Autodesk Fusion 360 part; units mm, degrees
sketch "Sketch1" plane through (0, 0, 0) normal (0, 1, 0) x (1, 0, 0)
  line L0 (0, 0) -> (50, 0)
  line L1 (50, 0) -> (50, -30)
  line L2 (50, -30) -> (0, -30)
  line L3 (0, -30) -> (0, 0)
  circle A0 centre (5.5, -15) radius 1.6
  circle A1 centre (44.5, -15) radius 1.6
  circle A2 centre (25, -21.15) radius 2.1
  point P0 (25, -21.15)
  dimension "d1" = 30
  dimension "d2" = 50
  dimension "d3" = 15
  dimension "d4" = 5.5
  dimension "d5" = 5.5
  dimension "d6" = 3.2
  dimension "d9" = 25
  dimension "d10" = 21.15
  dimension "d19" = 4.2
extrude "Extrude1" add sketch "Sketch1" against normal blind 5
sketch "Sketch2" plane through (0, -5, 0) normal (0, -1, 0) x (1, 0, 0)
  circle A0 centre (44.5, 15) radius 1.6
  circle A1 centre (5.5, 15) radius 1.6
  line L0 (50, 30) -> (0, 30)
  line L1 (0, 30) -> (0, 0)
  line L2 (0, 0) -> (50, 0)
  line L3 (50, 0) -> (50, 30)
  line L4 (33.75, 33.4) -> (16.25, 33.4)
  line L5 (16.25, 33.4) -> (16.25, 8.9)
  line L6 (16.25, 8.9) -> (33.75, 8.9)
  line L7 (33.75, 8.9) -> (33.75, 33.4)
  line L8 (33.75, 33.4) -> (16.25, 8.9) construction
  line L9 (16.25, 33.4) -> (33.75, 8.9) construction
  circle A2 centre (25, 21.15) radius 2.1
  line L10 (29.75, 12.9) -> (20.25, 12.9)
  line L11 (20.25, 12.9) -> (20.25, 29.4)
  line L12 (20.25, 29.4) -> (29.75, 29.4)
  line L13 (29.75, 29.4) -> (29.75, 12.9)
  line L14 (29.75, 12.9) -> (20.25, 29.4) construction
  line L15 (20.25, 12.9) -> (29.75, 29.4) construction
  point P0 (25, 21.15)
  point P1 (25, 21.15)
  dimension "d20" = 16.5
  dimension "d21" = 9.5
  dimension "d22" = 4
  dimension "d23" = 4
extrude "Extrude2" add sketch "Sketch2" along normal blind 14 and the other way up to surface (5 mm away) contours L0 L5 L6 L7 | L0 L4 L5 L7
extrude "Extrude3" cut 1 faces at (25.0523, -5, 14.952) along direction (0, 1, 0) blind 2
sketch "Sketch3" plane through (0, 0, 0) normal (0, 1, 0) x (-1, 0, 0)
  circle A0 centre (-5.5, 15) radius 1.6
  circle A1 centre (-44.5, 15) radius 1.6
  line L0 (-33.75, 30) -> (-50, 30)
  line L1 (-50, 30) -> (-50, 0)
  line L2 (-50, 0) -> (0, 0)
  line L3 (0, 0) -> (0, 30)
  line L4 (0, 30) -> (-16.25, 30)
  line L5 (-16.25, 30) -> (-16.25, 33.4)
  line L6 (-16.25, 33.4) -> (-33.75, 33.4)
  line L7 (-33.75, 33.4) -> (-33.75, 30)
  circle A2 centre (-25, 21.15) radius 2.1
  circle A3 centre (-44.5, 7) radius 3
  circle A4 centre (-5.5, 7) radius 3
  dimension "d28" = 6
  dimension "d32" = 8
extrude "Extrude4" cut sketch "Sketch3" against normal blind 3 contours A3 | A4
chamfer "Chamfer1" distance 8.9 angle 45 3 edges at (16.25, -5, 19.45) (33.75, -5, 19.45) (25, -5, 8.9)
chamfer "Chamfer3" distance 4 angle 45 2 edges at (33.75, -9.5, 33.4) (16.25, -9.5, 33.4)
fillet "Fillet2" radius 3 10 edges at (0, -2.5, 30) (0, -2.5, 0) (50, -2.5, 30) (50, -2.5, 0) (33.75, -16.45, 8.9) (16.25, -16.45, 8.9) (16.25, -16.45, 29.4) (20.25, -9.5, 33.4) (29.75, -9.5, 33.4) (33.75, -16.45, 29.4)
equation "d3 = d1 / 2"
equation "d5 = d4"
equation "d9 = d2 / 2"
equation "d10 = ( 42.3 / 2 ) * 1 mm"
equation "d23 = d22"
Model file for the job. Use its own axes, mm. A direction names the side the tool comes from. Coordinates: 2 decimals unless noted, no trailing zeros. Order: outer loops, then holes, each group sorted by start corner. A loop starts at its lowest first (then second) coordinate and runs counter-clockwise, first axis right, second up. Notation, with made-up numbers: (31, 5) -> (40, 5) arc R23 cw to (40, 26) -> close; hole circle Ø10 at (-9, -15). An arc over 180 degrees is marked (long way). Return JSON: item names as keys, results as strings. Group by question number.
Item 1: Wall check: line 1 along Z through (x, y) = (5.5, -1.1); line 2 along X through (y, z) = (-2.1, 15); line 3 along Z through (x, y) = (25, -1.65). Give the ranges that are in metal, low to high. Write a range as [from, to].
Item 2: Saw through at B-B on x = 44.5. Write the cut outline in (y, z).
Item 3: Saw through at C-C on z = 21.15. Write the cut outline in (x, y), then the cut area to 3 significant figures.
Item 4: Pull direction X, two halves, no side cores. Call faces 6 (the flat face through (12, -6, 30)), 7 (the cylindrical face through (33.453, -14.47, 29.46)), 8 (the cylindrical face through (47.5, -1.5, 7.1)): pulls with the +X half, pulls with the -X half, needs draft (parallel to the pull), parting line crosses it, or undercut.
Item 5: Flat gauge pins, fed straight in: P1, Ø3, axis at x = 23.5, z = 18.5, coming from the -Y side; P2, Ø1.8, axis at x = 4.5, z = 8, coming from the +Y side; P3, Ø10.5, axis at x = 25, y = -10.5, coming from the -Z side. Where does each tip first touch, or does it go through?
Item 6: Tool access for faces 1 (the flat face through (33.75, -16, 20)), 2 (the flat face through (6, -3, 7)), 3 (the flat face through (25, -16, 8.9)), 4 (the flat face through (29.75, -11, 21)), 5 (the cylindrical face through (16.51, -14.38, 29.38)): list every direction of +Z, -Z, +X, -X, +Y, -Y with a clear straight run to the whole face (end or side of a thin tool).
Item 7: Saw through at A-A on y = -17. Write the cut outline in (x, z).
Item 8: Saw through at D-D on y = -1.75. Write the cut outline in (x, z), then the cut area to 3 significant figures.
Values found:
{
 "1": {"line 1": "z = [0, 4], [10, 13.4], [16.6, 30]", "line 2": "x = [0, 3.9], [7.1, 42.9], [46.1, 50]", "line 3": "z = [0, 19.05], [23.25, 33.4]"},
 "2": {"outline": "(-5, 0) -> (0, 0) -> (0, 4) -> (-3, 4) -> (-3, 10) -> (0, 10) -> (0, 13.4) -> (-5, 13.4) -> close; (-5, 16.6) -> (0, 16.6) -> (0, 30) -> (-5, 30) -> close"},
 "3": {"outline": "(0, -5) -> (7.35, -5) -> (16.25, -13.9) -> (16.25, -19) -> (20.25, -19) -> (20.25, -3) -> (22.9, -3) -> (22.9, 0) -> (0, 0) -> close; (27.1, -3) -> (29.75, -3) -> (29.75, -19) -> (33.75, -19) -> (33.75, -13.9) -> (42.65, -5) -> (50, -5) -> (50, 0) -> (27.1, 0) -> close", "area": "410 mm2"},
 "4": {"face 6": "needs draft", "face 7": "pulls with the +X half", "face 8": "undercut"},
 "5": {"P1": "stops at y = -3", "P2": "stops at y = -3", "P3": "stops at z = 0.25"},
 "6": {"face 1": "+Z, -Z, +X, -Y", "face 2": "+Y", "face 3": "-Z, +X, -X, -Y", "face 4": "-Y", "face 5": "+Z, -X, -Y"},
 "7": {"outline": "(16.25, 11.9) arc R3 ccw to (19.25, 8.9) -> (30.75, 8.9) arc R3 ccw to (33.75, 11.9) -> (33.75, 28.16) arc R3 ccw to (32.87, 30.28) -> (30.63, 32.52) arc R3 ccw to (28.51, 33.4) -> (21.49, 33.4) arc R3 ccw to (19.37, 32.52) -> (17.13, 30.28) arc R3 ccw to (16.25, 28.16) -> close; hole (20.25, 12.9) -> (29.75, 12.9) -> (29.75, 29.4) -> (20.25, 29.4) -> close"},
 "8": {"outline": "(0, 3) arc R3 ccw to (3, 0) -> (47, 0) arc R3 ccw to (50, 3) -> (50, 27) arc R3 ccw to (47, 30) -> (33.12, 30) arc R3 ccw to (32.87, 30.28) -> (30.63, 32.52) arc R3 ccw to (28.51, 33.4) -> (21.49, 33.4) arc R3 ccw to (19.37, 32.52) -> (17.13, 30.28) arc R3 ccw to (16.88, 30) -> (3, 30) arc R3 ccw to (0, 27) -> close; hole circle Ø6 at (5.5, 7); hole circle Ø3.2 at (5.5, 15); hole circle Ø4.2 at (25, 21.15); hole circle Ø6 at (44.5, 7); hole circle Ø3.2 at (44.5, 15)", "area": "1,450 mm2"}
}
